Could you check a few things on this model? Use its own coordinates, in mm. A direction names the side the tool comes from. Give positions to 0.01 mm unless a question says otherwise; leave off trailing zeros. Loops run counter-clockwise (first coordinate to the right, second up) from the corner with the lowest first, then second, coordinate; pieces in that order, holes last. Notation, with made-up numbers: (-19.5, 18) - (4.5, 18) arc R21 cw to (4.5, 55) - close; hole circle Ø9 at (41.5, 33.5). An arc over 180 degrees is marked (long way). Answer in a Markdown table with one row per item. Add a question column.
```python
from build123d import *

# Parameters (mm, degrees)
SCHNITT_LINEAR_AUSTRAGEN1_DEPTH = 7
SCHNITT_LINEAR_AUSTRAGEN2_DEPTH = 5


with BuildPart() as part:
    # Skizze1 → Rotation17 (revolve)
    with BuildSketch(Plane.XY, mode=Mode.PRIVATE) as rotation17_sk:
        Polygon((168.152402442, 0), (168.152402442, 26.5), (169.152402442, 27.5), (184.152402442, 27.5), (212.152402442, 27.5), (212.152402442, 29), (213.152402442, 30), (267.152402442, 30), (267.152402442, 32.5), (273.152402442, 32.5), (273.152402442, 30), (285.152402442, 30), (285.152402442, 27.5), (297.652402442, 27.5), (316.152402442, 27.5), (317.152402442, 26.5), (317.152402442, 25), (331.652402442, 25), (334.152402442, 23.556624327), (334.152402442, 20), (393.152402442, 20), (394.152402442, 19), (394.152402442, 0), align=None)
    revolve(rotation17_sk.sketch.rotate(Axis((168.152402442, 0, 0), (1, 0, 0)), 90), axis=Axis((168.152402442, 0, 0), (1, 0, 0)))  # turned: the seam where the file's is

    # Skizze3 → Schnitt-Linear austragen1 (cut)
    with BuildSketch(Plane.XY.offset(30)):
        with BuildLine():
            Line((228.652402442, 9), (255.652402442, 9))
            ThreePointArc((255.652402442, 9), (264.652402442, 0), (255.652402442, -9))
            Line((255.652402442, -9), (228.652402442, -9))
            ThreePointArc((228.652402442, -9), (219.652402442, 0), (228.652402442, 9))
        make_face()
    extrude(amount=-SCHNITT_LINEAR_AUSTRAGEN1_DEPTH, mode=Mode.SUBTRACT)

    # Skizze4 → Schnitt-Linear austragen2 (cut)
    with BuildSketch(Plane.XY.offset(20)):
        with BuildLine():
            Line((343.152402442, 6), (376.152402442, 6))
            ThreePointArc((376.152402442, 6), (382.152402442, 0), (376.152402442, -6))
            Line((376.152402442, -6), (343.152402442, -6))
            ThreePointArc((343.152402442, -6), (337.152402442, 0), (343.152402442, 6))
        make_face()
    extrude(amount=-SCHNITT_LINEAR_AUSTRAGEN2_DEPTH, mode=Mode.SUBTRACT)

    # Skizze16 → Nut f_r DIN 472 - 55 x 2_ Sicherungsring (revolve, cut)
    with BuildSketch(Plane(origin=(168.152402442, 0, 0), x_dir=(0, 0, 1), z_dir=(0, -1, 0))):
        with BuildLine():
            Line((28.785, -7.15), (24.75, -7.15))
            Line((24.75, -7.15), (24.75, -5))
            Line((24.75, -5), (28.785, -5))
            ThreePointArc((28.785, -5), (28.937027958, -5.062972042), (29, -5.215))
            Line((29, -5.215), (29, -6.935))
            ThreePointArc((29, -6.935), (28.937027958, -7.087027958), (28.785, -7.15))
        make_face()
    revolve(axis=Axis((218.152402442, 0, 0), (-1, 0, 0)), mode=Mode.SUBTRACT)

    # Skizze18 → Nut für DIN 472 - 40 x 1.75, Sicherungsring für Bohrungen - Regelausf.1 (revolve, cut)
    with BuildSketch(Plane(origin=(168.152402442, 0, 0), x_dir=(0, 0, 1), z_dir=(0, -1, 0))):
        with BuildLine():
            Line((21.065, -217.75), (18, -217.75))
            Line((18, -217.75), (18, -215.9))
            Line((18, -215.9), (21.065, -215.9))
            ThreePointArc((21.065, -215.9), (21.195814755, -215.954185245), (21.25, -216.085))
            Line((21.25, -216.085), (21.25, -217.565))
            ThreePointArc((21.25, -217.565), (21.195814755, -217.695814755), (21.065, -217.75))
        make_face()
    revolve(axis=Axis((218.152402442, 0, 0), (-1, 0, 0)), mode=Mode.SUBTRACT)

    # Skizze20 → Nut f_r DIN 472 - 55 x 2_ Sicherungs 2 (revolve, cut)
    with BuildSketch(Plane(origin=(168.152402442, 0, 0), x_dir=(0, 0, 1), z_dir=(0, -1, 0))):
        with BuildLine():
            Line((28.785, -144), (24.75, -144))
            Line((24.75, -144), (24.75, -141.85))
            Line((24.75, -141.85), (28.785, -141.85))
            ThreePointArc((28.785, -141.85), (28.937027958, -141.912972042), (29, -142.065))
            Line((29, -142.065), (29, -143.785))
            ThreePointArc((29, -143.785), (28.937027958, -143.937027958), (28.785, -144))
        make_face()
    revolve(axis=Axis((218.152402442, 0, 0), (-1, 0, 0)), mode=Mode.SUBTRACT)


solid = part.part
```
(1) We'd pull the mould along X, two halves only. Please class faces 4 (the cylindrical face through (382.15, 0.13, 17.54)), 5 (the cylindrical face through (314.124, 24.397, 12.69)), 6 (the flat face through (317.152, -16, 20)): pulls with the +X half, pulls with the -X half, needs draft (parallel to the pull), parting line crosses it, or undercut.
(2) For pin 1 Ø3.5 at (x, y) = (351, 2) entering from +Z; pin 2 Ø8 at (y, z) = (19.5, 24.5) entering from +X; pin 3 Ø1.5 at (y, z) = (20.5, 0.5) entering from +X, each with a flat end and sliding along its axis, tell me the tip position at first contact or that it passes through.
(3) On a 3-axis mill with a long thin cutter (end or side, diameter ignored), from which of +Z, -Z, +X, -X, +Y, -Y can I reach the whole of each face in a straight line? I mean faces 1 (the cylindrical face through (193.469, 24.397, 12.69)), 2 (the cylindrical face through (324.504, -7.509, 23.846)), 3 (the cylindrical face through (311.06, 24.54, -3.22)). Say none if no direction works.
(4) Please list where these lines run through material, in increasing order: line 1 (X direction, y = -15.5, z = -11); line 2 (X direction, y = 16, z = 22); line 3 (X direction, y = -19.5, z = 8).
(5) I want a section at B-B on x = 235. Please give me the cut outline in (y, z).
(6) I want a section at A-A on x = 347.5. Please give me the cut outline in (y, z), then the cut area to 3 significant figures.
Reported:
| question | item | result |
|---|---|---|
| 1 | face 4 | undercut |
| 1 | face 5 | needs draft |
| 1 | face 6 | pulls with the +X half |
| 2 | pin 1 | z = 15 |
| 2 | pin 2 | x = 316.34 |
| 2 | pin 3 | x = 393.4 |
| 3 | face 1 | -X |
| 3 | face 2 | +X |
| 3 | face 3 | none |
| 4 | line 1 | 168.15 to 384.05, 385.9 to 394.15 |
| 4 | line 2 | 168.86 to 173.15, 175.3 to 310, 312.15 to 316.45 |
| 4 | line 3 | 168.15 to 334.15 |
| 5 | outline | (-9, 23) - (-9, 28.62) arc R30 ccw (long way) to (9, 28.62) - (9, 23) - close |
| 6 | outline | (-6, 15) - (-6, 19.08) arc R20 ccw (long way) to (6, 19.08) - (6, 15) - close |
| 6 | area | 1,200 mm² |
